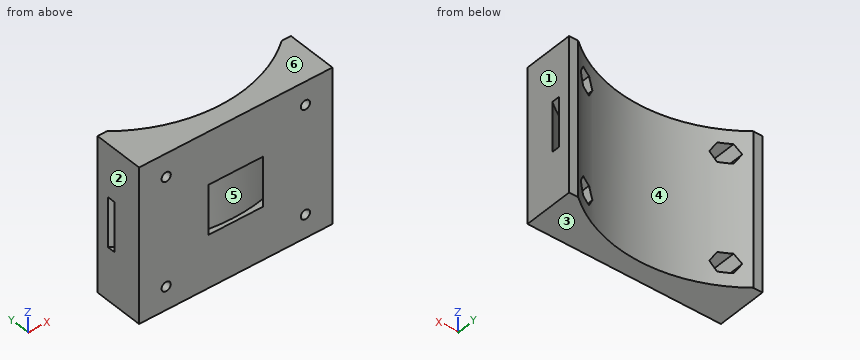
from build123d import *

# Parameters (mm, degrees)
BOSS_EXTRUDE1_DEPTH   = 63.5
SKETCH2_W             = 127
SKETCH2_H             = 12.7
CUT_EXTRUDE1_DEPTH    = 80.596939718
SKETCH3_W             = 20.32
SKETCH3_H             = 2.54
F_6_CLEARANCE_HOLE1_D = 3.7973
CUT_EXTRUDE2_DEPTH    = 22.225


with BuildPart() as part:
    # Sketch1 → Boss-Extrude1 (new body)
    with BuildSketch(Plane.XY):
        with BuildLine():
            Line((-39.6875, -3.022072464), (-39.6875, -26.9875))
            Line((-39.6875, -26.9875), (39.6875, -26.9875))
            Line((39.6875, -26.9875), (39.6875, -3.022072464))
            ThreePointArc((39.6875, -3.022072464), (0, -19.05), (-39.6875, -3.022072464))
        make_face()
    extrude(amount=BOSS_EXTRUDE1_DEPTH)

    # Sketch2 → Cut-Extrude1 (cut, through all)
    with BuildSketch(Plane.XY.offset(63.5)):
        Rectangle(SKETCH2_W, SKETCH2_H)
    extrude(amount=-CUT_EXTRUDE1_DEPTH, mode=Mode.SUBTRACT)

    # Sketch3 → Cut-Revolve1 (revolve, cut)
    with BuildSketch(Plane(origin=(0, 0, 0), x_dir=(0, 0, -1), z_dir=(1, 0, 0))):
        with Locations((-31.75, -26.67)):
            Rectangle(SKETCH3_W, SKETCH3_H)
    revolve(axis=Axis((0, 38.1, 16.404698597), (0, 0, 1)), mode=Mode.SUBTRACT)

    # #6 Clearance Hole1 (through all)
    with Locations(Plane(origin=(0, -26.9875, 0), x_dir=(-1, 0, 0), z_dir=(0, -1, 0))):
        with Locations((-28.575, -9.525), (-28.575, -53.975)):
            f_6_clearance_hole1 = Hole(F_6_CLEARANCE_HOLE1_D / 2)

    # Sketch10 → Cut-Extrude2 (cut)
    with BuildSketch(Plane(origin=(0, 0, 0), x_dir=(1, 0, 0), z_dir=(0, 1, 0))):
        Polygon((23.992282238, -9.525), (26.283641119, -13.49375), (30.866358881, -13.49375), (33.157717762, -9.525), (30.866358881, -5.55625), (26.283641119, -5.55625), align=None)
        Polygon((23.992282238, -53.975), (26.283641119, -57.94375), (30.866358881, -57.94375), (33.157717762, -53.975), (30.866358881, -50.00625), (26.283641119, -50.00625), align=None)
    cut_extrude2 = extrude(amount=-CUT_EXTRUDE2_DEPTH, mode=Mode.SUBTRACT)

    # Mirror1: #6 Clearance Hole1, Cut-Extrude2 across plane
    add(f_6_clearance_hole1.mirror(Plane(origin=(0, 0, 0), x_dir=(0, 0, 1), z_dir=(1, 0, 0))), mode=Mode.SUBTRACT)
    add(cut_extrude2.mirror(Plane(origin=(0, 0, 0), x_dir=(0, 0, 1), z_dir=(1, 0, 0))), mode=Mode.SUBTRACT)


solid = part.part
For this review, take the finished solid that the model builds, in its own axes (mm). Face numbers are marked on the shaded views. A direction names the side the tool comes from. Round coordinates to 2 decimals unless told otherwise and drop trailing zeros. Write each loop counter-clockwise with the first axis right and the second up, starting at its lowest first coordinate (ties: lowest second). Pieces come first, ordered by that corner, then holes. Notation, with made-up numbers: (87.5, 39) - (116.5, 39) arc R5 cw to (116.5, 45) - close; hole circle Ø11 at (89.25, 44.25). An arc over 180 degrees is marked (long way). Write item = value, one per line. Start each with the question number.
1. Consider section B-B on x = -28. State the section outline as (y, z) points (1 decimal).
2. Consider section C-C on x = 15. State the section outline as (y, z) points.
3. For the marked faces 5 and 6, list the 3-axis set-ups (+Z, -Z, +X, -X, +Y, -Y) from which the entire face can be reached by the end or side of a thin tool; tool diameter is ignored.
4. Wall thickness on L1, parallel to X at y = -26, z = 54; L2, parallel to Z at x = 28, y = -24.5; L3, parallel to Y at x = 1, z = 33: over which ranges is each line inside the solid? List them lowest first.
5. Consider section A-A on z = 32. State the section outline as (x, y) points.
6. Draft analysis for pull direction X (two halves, no side actions). For the marked faces 1, 2, 3 and 4, state which applies: released by +X, released by -X, zero draft, split by the parting line, or undercut.
7. For pin 1 Ø5 at (x, z) = (10.5, 34) entering from +Y; pin 2 Ø4.5 at (x, z) = (28.575, 53.975) entering from +Y (3 decimals); pin 3 Ø8.5 at (x, z) = (-29, 55.5) entering from +Y; pin 4 Ø5 at (x, y) = (28, -16.5) entering from -Z, all flat-tipped, find the tip position at first contact; note any pin that passes through.
Evaluation:
q1.outline = (-27, 0) - (-11.7, 0) - (-11.7, 5.6) - (-22.2, 5.6) - (-22.2, 7.7) - (-27, 7.7) - close; (-27, 11.3) - (-22.2, 11.3) - (-22.2, 13.5) - (-11.7, 13.5) - (-11.7, 50) - (-22.2, 50) - (-22.2, 52.2) - (-27, 52.2) - close; (-27, 55.8) - (-22.2, 55.8) - (-22.2, 57.9) - (-11.7, 57.9) - (-11.7, 63.5) - (-27, 63.5) - close; hole (-21.7, 21.6) - (-18.9, 21.6) - (-18.9, 41.9) - (-21.7, 41.9) - close
q2.outline = (-26.99, 0) - (-17.05, 0) - (-17.05, 63.5) - (-26.99, 63.5) - close; hole (-26.21, 21.59) - (-23.6, 21.59) - (-23.6, 41.91) - (-26.21, 41.91) - close
q3.face_5 = none
q3.face_6 = +Z, +X, -X, +Y, -Y
q4.L1 = -39.69 to -30.47, -26.68 to 26.68, 30.47 to 39.69
q4.L2 = 0 to 7.72, 11.33 to 52.17, 55.78 to 63.5
q4.L3 = -25.39 to -19.04
q5.outline = (-39.69, -26.99) - (-11.18, -26.99) arc R66.04 cw to (-39.69, -14.68) - close; (-39.69, -11.47) arc R63.5 ccw to (39.69, -11.47) - (39.69, -6.35) - (35.92, -6.35) arc R57.15 cw to (-35.92, -6.35) - (-39.69, -6.35) - close; (11.18, -26.99) - (39.69, -26.99) - (39.69, -14.68) arc R66.04 cw to start
q6.face_1 = released by +X
q6.face_2 = released by -X
q6.face_3 = zero draft
q6.face_4 = undercut
q7.pin_1 = -17.55
q7.pin_2 = -22.225
q7.pin_3 = -8.38
q7.pin_4 = 0
